from build123d import *

# Parameters (mm, degrees)
BOSS_EXTRUDE2_DEPTH         = 10.999999971
F_1_4_0_25_DIAMETER_HOLE1_D = 6.35
CUT_EXTRUDE1_DEPTH          = 42.363272981
F_1_4_20_TAPPED_HOLE1_D     = 5.1054


with BuildPart() as part:
    # Sketch2 → Boss-Extrude2 (new, symmetric)
    with BuildSketch(Plane.XY):
        with BuildLine():
            Line((-9.864999955, 19.999999846), (9.864999955, 19.999999846))
            ThreePointArc((9.864999955, 19.999999846), (10.314012761, 19.814012652), (10.499999955, 19.364999846))
            Line((10.499999955, 19.364999846), (10.499999955, 15.703539216))
            ThreePointArc((10.499999955, 15.703539216), (10.407835871, 15.025527914), (10.138031981, 14.396719989))
            Line((10.138031981, 14.396719989), (8.586360945, 11.810601618))
            ThreePointArc((8.586360945, 11.810601618), (8.241569778, 10.208887267), (8.946470225, 8.729872335))
            ThreePointArc((8.946470225, 8.729872335), (12.493042308, -0.417006435), (8.344414884, -9.307026416))
            ThreePointArc((8.344414884, -9.307026416), (7.720691236, -10.162643363), (7.499999986, -11.198214181))
            Line((7.499999986, -11.198214181), (7.499999986, -33.000000008))
            Line((7.499999986, -33.000000008), (8.690624986, -33.000000008))
            Line((8.690624986, -33.000000008), (8.690624986, -11.198214181))
            ThreePointArc((8.690624986, -11.198214181), (8.807867212, -10.648067184), (9.139220401, -10.193520681))
            ThreePointArc((9.139220401, -10.193520681), (13.683004586, -0.456726298), (9.798621513, 9.561392674))
            ThreePointArc((9.798621513, 9.561392674), (9.42414315, 10.347119357), (9.607313458, 11.198030105))
            Line((9.607313458, 11.198030105), (11.158984494, 13.784148477))
            ThreePointArc((11.158984494, 13.784148477), (11.555258957, 14.707710116), (11.690624955, 15.703539216))
            Line((11.690624955, 15.703539216), (11.690624955, 19.364999846))
            ThreePointArc((11.690624955, 19.364999846), (11.155911772, 20.655911664), (9.864999955, 21.190624846))
            Line((9.864999955, 21.190624846), (-9.864999955, 21.190624846))
            ThreePointArc((-9.864999955, 21.190624846), (-11.155911772, 20.655911664), (-11.690624955, 19.364999846))
            Line((-11.690624955, 19.364999846), (-11.690624955, 15.703539216))
            ThreePointArc((-11.690624955, 15.703539216), (-11.555258957, 14.707710116), (-11.158984494, 13.784148477))
            Line((-11.158984494, 13.784148477), (-9.607313458, 11.198030105))
            ThreePointArc((-9.607313458, 11.198030105), (-9.42414315, 10.347119357), (-9.798621513, 9.561392674))
            ThreePointArc((-9.798621513, 9.561392674), (-13.683004586, -0.456726298), (-9.139220401, -10.193520681))
            ThreePointArc((-9.139220401, -10.193520681), (-8.807867212, -10.648067184), (-8.690624986, -11.198214181))
            Line((-8.690624986, -11.198214181), (-8.690624986, -33.000000008))
            Line((-8.690624986, -33.000000008), (-7.499999986, -33.000000008))
            Line((-7.499999986, -33.000000008), (-7.499999986, -11.198214181))
            ThreePointArc((-7.499999986, -11.198214181), (-7.720691236, -10.162643363), (-8.344414884, -9.307026416))
            ThreePointArc((-8.344414884, -9.307026416), (-12.493042308, -0.417006435), (-8.946470225, 8.729872335))
            ThreePointArc((-8.946470225, 8.729872335), (-8.241569778, 10.208887267), (-8.586360945, 11.810601618))
            Line((-8.586360945, 11.810601618), (-10.138031981, 14.396719989))
            ThreePointArc((-10.138031981, 14.396719989), (-10.407835871, 15.025527914), (-10.499999955, 15.703539216))
            Line((-10.499999955, 15.703539216), (-10.499999955, 19.364999846))
            ThreePointArc((-10.499999955, 19.364999846), (-10.314012761, 19.814012652), (-9.864999955, 19.999999846))
        make_face()
    extrude(amount=BOSS_EXTRUDE2_DEPTH, both=True)

    # 1/4 (0.25) Diameter Hole1 (through all)
    with Locations(Plane(origin=(0, 21.190624846, 0), x_dir=(1, 0, 0), z_dir=(0, 1, 0))):
        with Locations((0, 0)):
            Hole(F_1_4_0_25_DIAMETER_HOLE1_D / 2)

    # Sketch6 → Cut-Extrude1 (cut, through all)
    with BuildSketch(Plane(origin=(8.690624986, 0, 0), x_dir=(0, 0, -1), z_dir=(1, 0, 0))):
        with BuildLine():
            Line((-10.999999971, -33.000000008), (0, -33.000000008))
            ThreePointArc((0, -33.000000008), (-5.640257081, -32.367131167), (-10.999999971, -30.499999928))
            Line((-10.999999971, -30.499999928), (-10.999999971, -33.000000008))
        make_face()
        with BuildLine():
            Line((0, -33.000000008), (10.999999971, -33.000000008))
            Line((10.999999971, -33.000000008), (10.999999971, -30.499999928))
            ThreePointArc((10.999999971, -30.499999928), (5.640257081, -32.367131167), (0, -33.000000008))
        make_face()
    extrude(amount=-CUT_EXTRUDE1_DEPTH, mode=Mode.SUBTRACT)

    # 1/4-20 Tapped Hole1 (through all)
    with Locations(Plane(origin=(8.690624986, -25.380000008, 0), x_dir=(0, 1, 0), z_dir=(1, 0, 0))):
        with Locations((0, 0)):
            Hole(F_1_4_20_TAPPED_HOLE1_D / 2)


solid = part.part
Can you work these out from the model? Positions are in its coordinate system, mm. A direction names the side the tool comes from. Round coordinates to 2 decimals unless told otherwise and drop trailing zeros. Loops run counter-clockwise (first coordinate to the right, second up) from the corner with the lowest first, then second, coordinate; pieces in that order, holes last. Notation, with made-up numbers: (61, 47) - (105, 47) arc R34 cw to (105, 86) - close; hole circle Ø11 at (81, 16). An arc over 180 degrees is marked (long way). Write item = value, one per line. Start each with the question number.
(1) If we mould it in two halves opening along Z, with no side actions, what happens to faces 5 (the face through (-9, 9, 11)), 6 (the face through (-8.104, -27.738, -0.978)), 7 (the face through (-8.244, 10.186, 0.154))? For each: released by +Z, released by -Z, zero draft, split by the parting line, or undercut.
(2) If we section it at D-D (x = 6.75): Please give me the cut outline in (y, z), and give its area (3 significant figures).
(3) If we section it at B-B (y = 0): Please give me the cut outline in (x, z).
(4) For P1, Ø3, axis at y = -6.5, z = 8.5, coming from the +X side; P2, Ø1.8, axis at y = 17, z = 5.5, coming from the -X side; P3, Ø10, axis at x = 0, z = 0, coming from the -Y side; P4, Ø4, axis at y = -25.38, z = 0, coming from the +X side, each with a flat end and sliding along its axis, tell me the tip position at first contact or that it passes through.
(5) If I drill on probe 1 along Z at (x, y) = (7.9, -25.38); probe 2 along Y at (x, z) = (7.75, 0.5); probe 3 along Z at (x, y) = (0, 20.3) (3 decimals), over which ranges is the centre line in solid material (lowest first)? Write a range as [from, to].
(6) If we section it at C-C (y = -25.38): Please give me the cut outline in (x, z), and give its area (3 significant figures).
(7) For faces 1 (the face through (-9.351, 13.086, 0.154)), 2 (the face through (11.55, 14.69, 0.15)), 3 (the face through (-9, 9, -11)), 4 (the face through (-8.691, -22, 0)), which set-ups out of +Z, -Z, +X, -X, +Y, -Y let a thin tool reach every point of the face, with its end or its side?
(8) If we section it at A-A (x = 0): Please give me the cut outline in (y, z) (3 decimals), and give its area (3 significant figures).
Ans:
q1.face_5 = released by +Z
q1.face_6 = undercut
q1.face_7 = zero draft
q2.outline = (20, -11) - (21.19, -11) - (21.19, 11) - (20, 11) - close
q2.area = 26.2 mm²
q3.outline = (-13.69, -11) - (-12.5, -11) - (-12.5, 11) - (-13.69, 11) - close; (12.5, -11) - (13.69, -11) - (13.69, 11) - (12.5, 11) - close
q4.P1 = 12.74
q4.P2 = -11.69
q4.P3 = 20
q4.P4 = through
q5.probe_1 = [-11, -2.55], [2.55, 11]
q5.probe_2 = [-33, -27.88], [-22.88, -10.1], [20, 21.19]
q5.probe_3 = [-11, -3.175], [3.175, 11]
q6.outline = (-8.69, -11) - (-7.5, -11) - (-7.5, -2.55) - (-8.69, -2.55) - close; (-8.69, 2.55) - (-7.5, 2.55) - (-7.5, 11) - (-8.69, 11) - close; (7.5, -11) - (8.69, -11) - (8.69, -2.55) - (7.5, -2.55) - close; (7.5, 2.55) - (8.69, 2.55) - (8.69, 11) - (7.5, 11) - close
q6.area = 40.2 mm²
q7.face_1 = +Z, -Z
q7.face_2 = +Z, -Z, +X
q7.face_3 = -Z, +X, -X, +Y, -Y
q7.face_4 = +Z, -Z, -X, -Y
q8.outline = (20, -11) - (21.191, -11) - (21.191, -3.175) - (20, -3.175) - close; (20, 3.175) - (21.191, 3.175) - (21.191, 11) - (20, 11) - close
q8.area = 18.6 mm²
